Input: part model. Units: mm. Frame: model coordinates. Face numbers are marked on the shaded views. A direction names the side the tool comes from. Give positions to 0.01 mm unless a question says otherwise; leave off trailing zeros. Order: outer loops, then holes, each group sorted by start corner. A loop starts at its lowest first (then second) coordinate and runs counter-clockwise, first axis right, second up. Notation, with made-up numbers: (30.25, 47) - (89.25, 47) arc R20 ccw to (89.25, 53) - close; hole circle Ø5 at (-36, 65.25). An arc over 180 degrees is marked (long way). Answer in a Markdown table with one row per item. Add a question column.
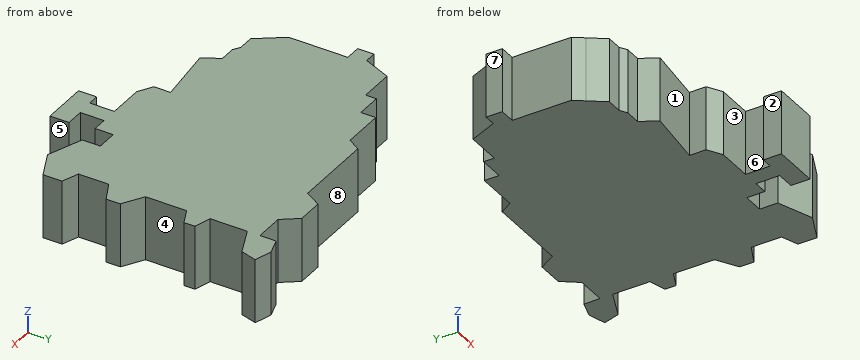
from build123d import *

# Parameters (mm, degrees)
F1_DEPTH = 25.4


with BuildPart() as f1:
    # F0 (on Top) → F1 (new body)
    with BuildSketch(Plane.XY):
        Polygon((-61.666694, -3.410565), (-55.360642, -3.410565), (-55.360642, -26.823629), (-52.448954, -30.879436), (-47.840081, -37.299322), (-41.626241, -37.299322), (-38.806695, -38.991049), (-32.53863, -38.991049), (-28.851533, -45.627825), (-5.598422, -42.862501), (-5.598422, -49.458609), (0, -52.817661), (14.2875, -52.817661), (14.2875, -62.588468), (9.862985, -62.588468), (9.862985, -69.778308), (28.114116, -69.778308), (28.114116, -62.219758), (20.924276, -62.219758), (20.924276, -52.817661), (26.639272, -52.817661), (26.639272, -45.627825), (34.93524, -45.627825), (34.93524, -52.817661), (48.761852, -57.979599), (60.007501, -52.817661), (60.007501, -45.259114), (53.370729, -42.862501), (53.370729, -30.879436), (61.558252, -26.823629), (61.558252, -21.227917), (53.370729, -16.315404), (53.370729, 0), (60.007501, 3.041855), (60.007501, 7.466371), (53.370729, 9.30992), (53.370729, 24.058307), (64.910345, 29.035889), (66.828631, 35.488307), (60.007501, 37.51621), (53.370729, 35.488307), (53.370729, 29.035889), (41.756369, 29.035889), (36.963142, 35.488307), (26.639272, 35.488307), (22.767821, 29.035889), (-9.30992, 29.035889), (-12.443951, 24.058307), (-28.851533, 24.058307), (-28.851533, 18.158952), (-38.806695, 18.158952), (-38.806695, 13.91879), (-52.448954, 13.91879), (-57.057824, 3.041855), (-61.666694, 3.041855), (-61.666694, 0), align=None)
    extrude(amount=F1_DEPTH)


solid = f1.part
Q1. Pull-direction query (Y, two-part tool) for the marked faces 6, 7 and 8; classes: +Y half, -Y half, draft (parallel to the pull), parting line (faces both ways), or undercut.
Q2. Section C-C, the plane x = 44. Return loops of the section in (y, z), then the cut area to 3 significant figures.
Q3. Line query: probe 1 along X at (y, z) = (-46, 5.5); probe 2 along Y at (x, z) = (27.5, 5.5); probe 3 along Y at (x, z) = (54, 20.5). Output: solid intervals per line, ascending.
Q4. Section B-B, the plane y = -25. Return loops of the section in (x, z).
Q5. Section A-A, the plane x = 12. Return loops of the section in (y, z), then the cut area to 3 significant figures.
Q6. Contact query for flat-ended pins moving along their axis: P1, Ø8, axis at y = -34, z = 19, coming from the -X side; P2, Ø3.5, axis at y = 5, z = 9.5, coming from the +X side; P3, Ø3, axis at y = 21, z = 9.5, coming from the -X side; P4, Ø10, axis at x = -17, y = -50, coming from the -Z side. Output: stop coordinate, or through.
Q7. Access query for the marked faces 1, 2, 3, 4 and 5. Directions: +Z, -Z, +X, -X, +Y, -Y. A direction counts if a zero-diameter tool reaches every point of the face in a straight line with its end or side. Return the directions, or none.
Computed:
| question | item | result |
|---|---|---|
| 1 | face 6 | undercut |
| 1 | face 7 | draft |
| 1 | face 8 | +Y half |
| 2 | outline | (-56.2, 0) - (29.04, 0) - (29.04, 25.4) - (-56.2, 25.4) - close |
| 2 | area | 2,170 mm^2 |
| 3 | probe 1 | x = -5.6 to 26.64, 34.94 to 60.01 |
| 3 | probe 2 | y = -69.78 to -62.22, -45.63 to 35.49 |
| 3 | probe 3 | y = -55.58 to -43.09, -30.57 to -16.69, 0.29 to 9.14, 24.33 to 35.68 |
| 4 | outline | (-55.36, 0) - (61.56, 0) - (61.56, 25.4) - (-55.36, 25.4) - close |
| 5 | outline | (-69.78, 0) - (-62.59, 0) - (-62.59, 25.4) - (-69.78, 25.4) - close; (-52.82, 0) - (29.04, 0) - (29.04, 25.4) - (-52.82, 25.4) - close |
| 5 | area | 2,260 mm^2 |
| 6 | P1 | stops at x = -53.08 |
| 6 | P2 | stops at x = 60.01 |
| 6 | P3 | stops at x = -28.85 |
| 6 | P4 | passes through |
| 7 | face 1 | +Z, -Z, -Y |
| 7 | face 2 | +Z, -Z, -X, -Y |
| 7 | face 3 | +Z, -Z, -X |
| 7 | face 4 | +Z, -Z, +X |
| 7 | face 5 | +Z, -Z, +X, -Y |
